For this review, take the finished solid that the model builds, in its own axes (mm). A direction names the side the tool comes from. Round coordinates to 2 decimals unless told otherwise and drop trailing zeros. Order: outer loops, then holes, each group sorted by start corner. A loop starts at its lowest first (then second) coordinate and runs counter-clockwise, first axis right, second up. Notation, with made-up numbers: M 29,33 L 70,33 A17 cw 70,41 Z; hole C -33.5,9.5 d5. An arc over 180 degrees is marked long. Put each result on its own line as item: value.
from build123d import *

# Parameters (mm, degrees)
ESQUISSE1_W             = 450
ESQUISSE1_H             = 15.25
BOSS_EXTRU_1_DEPTH      = 300
ESQUISSE2_W             = 17.25
ESQUISSE2_H             = 300
ENL_V_MAT_EXTRU_1_DEPTH = 8.625
ENL_V_MAT_EXTRU_2_REACH = 17.25
ESQUISSE3_R             = 40
ESQUISSE3_R_2           = 20


with BuildPart() as part:
    # Esquisse1 → Boss.-Extru.1 (new body)
    with BuildSketch(Plane.XY):
        with Locations((-225, 52.688864629)):
            Rectangle(ESQUISSE1_W, ESQUISSE1_H)
    extrude(amount=BOSS_EXTRU_1_DEPTH)

    # Esquisse2 → Enlèv. mat.-Extru.1 (cut)
    with BuildSketch(Plane(origin=(0, 60.313864629, 0), x_dir=(1, 0, 0), z_dir=(0, 1, 0))):
        with Locations((-307.625, -150)):
            Rectangle(ESQUISSE2_W, ESQUISSE2_H)
    extrude(amount=-ENL_V_MAT_EXTRU_1_DEPTH, mode=Mode.SUBTRACT)

    # Esquisse3 → Enlèv. mat.-Extru.2 (cut, up to next)
    with BuildSketch(Plane(origin=(0, 60.313864629, 0), x_dir=(1, 0, 0), z_dir=(0, 1, 0)), mode=Mode.PRIVATE) as enl_v_mat_extru_2_sk1:
        with Locations((-150, -140.161341078)):
            Circle(ESQUISSE3_R)
    enl_v_mat_extru_2_tool1 = extrude(enl_v_mat_extru_2_sk1.sketch, amount=-ENL_V_MAT_EXTRU_2_REACH, mode=Mode.PRIVATE) & part.part
    add(enl_v_mat_extru_2_tool1.solids().sort_by_distance((-150, 60.313865, 140.161341))[0], mode=Mode.SUBTRACT)
    # Esquisse3 → Enlèv. mat.-Extru.2 (cut, up to next)
    with BuildSketch(Plane(origin=(0, 60.313864629, 0), x_dir=(1, 0, 0), z_dir=(0, 1, 0)), mode=Mode.PRIVATE) as enl_v_mat_extru_2_sk2:
        with Locations((-383.125, -140.161341078)):
            Circle(ESQUISSE3_R_2)
    enl_v_mat_extru_2_tool2 = extrude(enl_v_mat_extru_2_sk2.sketch, amount=-ENL_V_MAT_EXTRU_2_REACH, mode=Mode.PRIVATE) & part.part
    add(enl_v_mat_extru_2_tool2.solids().sort_by_distance((-383.125, 60.313865, 140.161341))[0], mode=Mode.SUBTRACT)


solid = part.part
(1) Add section A-A on y = 57. Give the boundary of the cut face in (x, z) (3 decimals).
A:
outline: M -450,0 L -316.25,0 L -316.25,300 L -450,300 Z; M -299,0 L 0,0 L 0,300 L -299,300 Z; hole C -383.125,140.161 d40; hole C -150,140.161 d80
(2) Add section C-C on z = 266.5. Give the boundary of the cut face in (x, y).
A:
outline: M -450,45.06 L 0,45.06 L 0,60.31 L -299,60.31 L -299,51.69 L -316.25,51.69 L -316.25,60.31 L -450,60.31 Z
(3) Draft analysis for pull direction Z (two halves, no side actions). For faces 1 (the face through (-228, 53, 0)), 2 (the face through (-308, 51.689, 148)), 3 (the face through (-364.05, 52.8, 134.15)), state which applies: released by +Z, released by -Z, zero draft, split by the parting line, or undercut.
A:
face 1: released by -Z
face 2: zero draft
face 3: undercut
(4) Add section B-B on x = -150. Give the boundary of the cut face in (y, z).
A:
outline: M 45.06,0 L 60.31,0 L 60.31,100.16 L 45.06,100.16 Z; M 45.06,180.16 L 60.31,180.16 L 60.31,300 L 45.06,300 Z
(5) For faces 4 (the face through (-450, 53, 148)), 5 (the face through (-299, 56, 152)), list the 3-axis set-ups (+Z, -Z, +X, -X, +Y, -Y) from which the entire face can be reached by the end or side of a thin tool; tool diameter is ignored.
A:
face 4: +Z, -Z, -X, +Y, -Y
face 5: +Z, -Z, +Y
(6) To check wall thickness, follow L1, parallel to X at y = 58.25, z = 171.5; L2, parallel to Z at x = -150, y = 50.75; L3, parallel to X at y = 57, z = 205. State the ranges of each line that lie inside material, in increasing order.
A:
L1: x = -450 to -316.25, -299 to -174.86, -125.14 to 0
L2: z = 0 to 100.16, 180.16 to 300
L3: x = -450 to -316.25, -299 to 0
